Study the drawing (mm; zero at the part's minimum x, y, z) and answer. A direction names the side the tool comes from. Coordinates: 2 decimals unless noted, no trailing zeros. Loops run counter-clockwise (first coordinate to the right, second up) from the corner with the lowest first, then second, coordinate; pieces in that order, holes last.
Q1. The mould has two halves that part along X. Classify the marked faces 1, 2, 3 and 4: pulls with the +X half, pulls with the -X half, needs draft (parallel to the pull), parting line crosses it, or undercut.
Q2. Straight lines are drawn through the part: line 1 (X direction, y = 13.5, z = 14.5); line 2 (Z direction, x = 32.5, y = 23); line 3 (Z direction, x = 18, y = 19.75). For each, find the intervals that lie inside material, in ascending order.
Q3. Section A-A (x = 32.5) is taken. Give the vertices of the cut face in (y, z), then the cut area to 3 significant figures.
Q4. Flat-ended cylindrical pins translate along their axes: P1, Ø2, axis at x = 34, z = 25.5, coming from the -Y side; P2, Ø4, axis at x = 27.5, y = 21, coming from the +Z side; P3, Ø11, axis at x = 33, y = 12, coming from the +Z side; P4, Ø1, axis at y = 4.5, z = 35, coming from the -X side. Find the tip coordinate at first contact, or state that the pin passes through.
Q5. Section D-D (x = 17) is taken. Give the vertices of the cut face in (y, z), then the cut area to 3 significant figures.
Q6. Section C-C (z = 11) is taken. Give the vertices of the cut face in (x, y) (1 decimal).
Q7. Which of the six approach directions +Z, -Z, +X, -X, +Y, -Y give full straight-line access (tool end or side, diameter ignored) to the marked faces 5, 6, 7, 8 and 9?
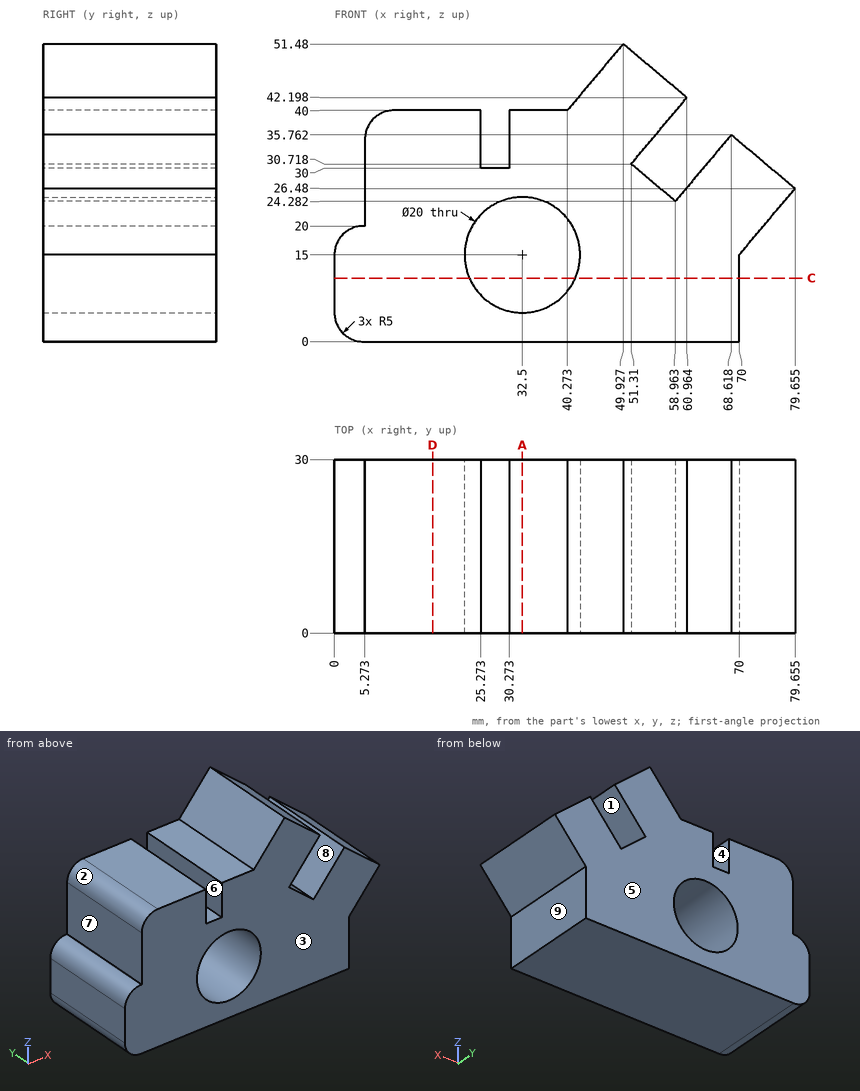
Numbers:
1. face 1: undercut
1. face 2: pulls with the -X half
1. face 3: needs draft
1. face 4: undercut
2. line 1: x = 0 to 22.51, 42.49 to 70
2. line 2: z = 0 to 5, 25 to 40
2. line 3: z = 0 to 40
3. outline: (0, 0) - (30, 0) - (30, 5) - (0, 5) - close; (0, 25) - (30, 25) - (30, 40) - (0, 40) - close
3. area: 600 mm2
4. P1: stops at y = 0
4. P2: stops at z = 30
4. P3: stops at z = 40
4. P4: stops at x = 5.27
5. outline: (0, 0) - (30, 0) - (30, 40) - (0, 40) - close
5. area: 1,200 mm2
6. outline: (0, 0) - (23.3, 0) - (23.3, 30) - (0, 30) - close; (41.7, 0) - (70, 0) - (70, 30) - (41.7, 30) - close
7. face 5: +Z, -Z, +X, -X, +Y
7. face 6: +Z, +Y, -Y
7. face 7: +Z, -X, +Y, -Y
7. face 8: +Y, -Y
7. face 9: -Z, +X, +Y, -Y
